```python
from build123d import *

# Parameters (mm, degrees)
EXTRUDE_1_DEPTH     = 4
EXTRUDE_2_DEPTH     = 8
CUT_EXTRUDE_1_DEPTH = 4


with BuildPart() as part:
    # Эскиз1 → Бобышка-Вытянуть1 (new body)
    with BuildSketch(Plane(origin=(0, 0, 0), x_dir=(0, 0, -1), z_dir=(1, 0, 0))):
        with BuildLine():
            Line((-7.553494652, -10.580393119), (-7.992649685, -0.342857143))
            ThreePointArc((-7.992649685, -0.342857143), (-0.171467962, 7.99816221), (8, 0))
            ThreePointArc((8, 0), (7.99816221, -0.171467962), (7.992649685, -0.342857143))
            Line((7.992649685, -0.342857143), (7.553494652, -10.580393119))
            ThreePointArc((7.553494652, -10.580393119), (11.428263628, -6.196352996), (12.988055737, -0.557142857))
            ThreePointArc((12.988055737, -0.557142857), (12.997013591, -0.278635438), (13, 0))
            ThreePointArc((13, 0), (-0.278635438, 12.997013591), (-12.988055737, -0.557142857))
            ThreePointArc((-12.988055737, -0.557142857), (-11.428263628, -6.196352996), (-7.553494652, -10.580393119))
        make_face()
        with BuildLine():
            Line((-4.727763281, -6.453545875), (-4.995406053, -0.214285714))
            ThreePointArc((-4.995406053, -0.214285714), (-0.107167476, 4.998851381), (5, 0))
            ThreePointArc((5, 0), (4.998851381, -0.107167476), (4.995406053, -0.214285714))
            Line((4.995406053, -0.214285714), (4.727763281, -6.453545875))
            ThreePointArc((4.727763281, -6.453545875), (7.056015568, -3.769966087), (7.992649685, -0.342857143))
            ThreePointArc((7.992649685, -0.342857143), (7.99816221, -0.171467962), (8, 0))
            ThreePointArc((8, 0), (-0.171467962, 7.99816221), (-7.992649685, -0.342857143))
            ThreePointArc((-7.992649685, -0.342857143), (-7.056015568, -3.769966087), (-4.727763281, -6.453545875))
        make_face()
        with BuildLine():
            Line((0, -8), (0, -5))
            ThreePointArc((0, -5), (-3.458942861, -3.610500559), (-4.995406053, -0.214285714))
            Line((-4.995406053, -0.214285714), (-4.727763281, -6.453545875))
            ThreePointArc((-4.727763281, -6.453545875), (-2.487130174, -7.603563868), (0, -8))
        make_face()
        with BuildLine():
            ThreePointArc((4.995406053, -0.214285714), (3.458942861, -3.610500559), (0, -5))
            Line((0, -5), (0, -8))
            ThreePointArc((0, -8), (2.487130174, -7.603563868), (4.727763281, -6.453545875))
            Line((4.727763281, -6.453545875), (4.995406053, -0.214285714))
        make_face()
        with BuildLine():
            ThreePointArc((4.727763281, -6.453545875), (2.487130174, -7.603563868), (0, -8))
            Line((0, -8), (0, -13))
            ThreePointArc((0, -13), (2.275699548, -12.799265274), (4.481120339, -12.203260241))
            Line((4.481120339, -12.203260241), (4.727763281, -6.453545875))
        make_face()
        with BuildLine():
            ThreePointArc((7.992649685, -0.342857143), (7.056015568, -3.769966087), (4.727763281, -6.453545875))
            Line((4.727763281, -6.453545875), (4.481120339, -12.203260241))
            ThreePointArc((4.481120339, -12.203260241), (6.071771893, -11.494937411), (7.553494652, -10.580393119))
            Line((7.553494652, -10.580393119), (7.992649685, -0.342857143))
        make_face()
        with BuildLine():
            Line((0, -13), (0, -8))
            ThreePointArc((0, -8), (-2.487130174, -7.603563868), (-4.727763281, -6.453545875))
            Line((-4.727763281, -6.453545875), (-4.481120339, -12.203260241))
            ThreePointArc((-4.481120339, -12.203260241), (-2.275699548, -12.799265274), (0, -13))
        make_face()
        with BuildLine():
            Line((-4.481120339, -12.203260241), (-4.727763281, -6.453545875))
            ThreePointArc((-4.727763281, -6.453545875), (-7.056015568, -3.769966087), (-7.992649685, -0.342857143))
            Line((-7.992649685, -0.342857143), (-7.553494652, -10.580393119))
            ThreePointArc((-7.553494652, -10.580393119), (-6.071771893, -11.494937411), (-4.481120339, -12.203260241))
        make_face()
        with BuildLine():
            Line((-3.966260715, -24.205613684), (-4.481120339, -12.203260241))
            ThreePointArc((-4.481120339, -12.203260241), (-6.071771893, -11.494937411), (-7.553494652, -10.580393119))
            Line((-7.553494652, -10.580393119), (-6.900606425, -25.80045485))
            ThreePointArc((-6.900606425, -25.80045485), (-5.491637274, -24.895945366), (-3.966260715, -24.205613684))
        make_face()
        with BuildLine():
            Line((-6.900606425, -25.80045485), (-7.553494652, -10.580393119))
            ThreePointArc((-7.553494652, -10.580393119), (-11.428263628, -6.196352996), (-12.988055737, -0.557142857))
            Line((-12.988055737, -0.557142857), (-11.489433922, -35.492857143))
            ThreePointArc((-11.489433922, -35.492857143), (-10.393943503, -30.07903074), (-6.900606425, -25.80045485))
        make_face()
        with BuildLine():
            Line((0, -23.5), (0, -13))
            ThreePointArc((0, -13), (-2.275699548, -12.799265274), (-4.481120339, -12.203260241))
            Line((-4.481120339, -12.203260241), (-3.966260715, -24.205613684))
            ThreePointArc((-3.966260715, -24.205613684), (-2.014268771, -23.677777545), (0, -23.5))
        make_face()
        with BuildLine():
            ThreePointArc((4.481120339, -12.203260241), (2.275699548, -12.799265274), (0, -13))
            Line((0, -13), (0, -23.5))
            ThreePointArc((0, -23.5), (2.014268771, -23.677777545), (3.966260715, -24.205613684))
            Line((3.966260715, -24.205613684), (4.481120339, -12.203260241))
        make_face()
        with BuildLine():
            ThreePointArc((7.553494652, -10.580393119), (6.071771893, -11.494937411), (4.481120339, -12.203260241))
            Line((4.481120339, -12.203260241), (3.966260715, -24.205613684))
            ThreePointArc((3.966260715, -24.205613684), (5.491637274, -24.895945366), (6.900606425, -25.80045485))
            Line((6.900606425, -25.80045485), (7.553494652, -10.580393119))
        make_face()
        with BuildLine():
            ThreePointArc((12.988055737, -0.557142857), (11.428263628, -6.196352996), (7.553494652, -10.580393119))
            Line((7.553494652, -10.580393119), (6.900606425, -25.80045485))
            ThreePointArc((6.900606425, -25.80045485), (10.286082196, -29.857382665), (11.5, -35))
            ThreePointArc((11.5, -35), (11.497358177, -35.246485195), (11.489433922, -35.492857143))
            Line((11.489433922, -35.492857143), (12.988055737, -0.557142857))
        make_face()
        with BuildLine():
            ThreePointArc((11.5, -35), (10.286082196, -29.857382665), (6.900606425, -25.80045485))
            Line((6.900606425, -25.80045485), (6.494027869, -35.278571429))
            ThreePointArc((6.494027869, -35.278571429), (0, -41.5), (-6.494027869, -35.278571429))
            Line((-6.494027869, -35.278571429), (-6.900606425, -25.80045485))
            ThreePointArc((-6.900606425, -25.80045485), (-10.393943503, -30.07903074), (-11.489433922, -35.492857143))
            ThreePointArc((-11.489433922, -35.492857143), (0, -46.5), (11.489433922, -35.492857143))
            ThreePointArc((11.489433922, -35.492857143), (11.497358177, -35.246485195), (11.5, -35))
        make_face()
        with BuildLine():
            ThreePointArc((6.5, -35), (5.766493566, -32.000408036), (3.731522476, -29.677806842))
            Line((3.731522476, -29.677806842), (3.496784237, -35.15))
            ThreePointArc((3.496784237, -35.15), (0, -38.5), (-3.496784237, -35.15))
            Line((-3.496784237, -35.15), (-3.731522476, -29.677806842))
            ThreePointArc((-3.731522476, -29.677806842), (-5.829460606, -32.124693225), (-6.494027869, -35.278571429))
            ThreePointArc((-6.494027869, -35.278571429), (0, -41.5), (6.494027869, -35.278571429))
            ThreePointArc((6.494027869, -35.278571429), (6.498506796, -35.139317719), (6.5, -35))
        make_face()
        with BuildLine():
            Line((-3.731522476, -29.677806842), (-3.966260715, -24.205613684))
            ThreePointArc((-3.966260715, -24.205613684), (-5.491637274, -24.895945366), (-6.900606425, -25.80045485))
            Line((-6.900606425, -25.80045485), (-6.494027869, -35.278571429))
            ThreePointArc((-6.494027869, -35.278571429), (-5.829460606, -32.124693225), (-3.731522476, -29.677806842))
        make_face()
        with BuildLine():
            Line((0, -28.5), (0, -23.5))
            ThreePointArc((0, -23.5), (-2.014268771, -23.677777545), (-3.966260715, -24.205613684))
            Line((-3.966260715, -24.205613684), (-3.731522476, -29.677806842))
            ThreePointArc((-3.731522476, -29.677806842), (-1.956494885, -28.801441477), (0, -28.5))
        make_face()
        with BuildLine():
            ThreePointArc((3.966260715, -24.205613684), (2.014268771, -23.677777545), (0, -23.5))
            Line((0, -23.5), (0, -28.5))
            ThreePointArc((0, -28.5), (1.956494885, -28.801441477), (3.731522476, -29.677806842))
            Line((3.731522476, -29.677806842), (3.966260715, -24.205613684))
        make_face()
        with BuildLine():
            Line((0, -31.5), (0, -28.5))
            ThreePointArc((0, -28.5), (-1.956494885, -28.801441477), (-3.731522476, -29.677806842))
            Line((-3.731522476, -29.677806842), (-3.496784237, -35.15))
            ThreePointArc((-3.496784237, -35.15), (-2.527350391, -32.578739997), (0, -31.5))
        make_face()
        with BuildLine():
            ThreePointArc((3.731522476, -29.677806842), (1.956494885, -28.801441477), (0, -28.5))
            Line((0, -28.5), (0, -31.5))
            ThreePointArc((0, -31.5), (2.474873734, -32.525126266), (3.5, -35))
            ThreePointArc((3.5, -35), (3.499195967, -35.075017233), (3.496784237, -35.15))
            Line((3.496784237, -35.15), (3.731522476, -29.677806842))
        make_face()
        with BuildLine():
            ThreePointArc((6.900606425, -25.80045485), (5.491637274, -24.895945366), (3.966260715, -24.205613684))
            Line((3.966260715, -24.205613684), (3.731522476, -29.677806842))
            ThreePointArc((3.731522476, -29.677806842), (5.766493566, -32.000408036), (6.5, -35))
            ThreePointArc((6.5, -35), (6.498506796, -35.139317719), (6.494027869, -35.278571429))
            Line((6.494027869, -35.278571429), (6.900606425, -25.80045485))
        make_face()
    extrude(amount=EXTRUDE_1_DEPTH)

    # Эскиз1<5> → Бобышка-Вытянуть2 (add)
    with BuildSketch(Plane(origin=(0, 0, 0), x_dir=(0, 0, -1), z_dir=(1, 0, 0))):
        with BuildLine():
            Line((-6.900606425, -25.80045485), (-7.553494652, -10.580393119))
            ThreePointArc((-7.553494652, -10.580393119), (-11.428263628, -6.196352996), (-12.988055737, -0.557142857))
            Line((-12.988055737, -0.557142857), (-11.489433922, -35.492857143))
            ThreePointArc((-11.489433922, -35.492857143), (-10.393943503, -30.07903074), (-6.900606425, -25.80045485))
        make_face()
        with BuildLine():
            Line((-6.494027869, -35.278571429), (-6.900606425, -25.80045485))
            ThreePointArc((-6.900606425, -25.80045485), (-10.393943503, -30.07903074), (-11.489433922, -35.492857143))
            ThreePointArc((-11.489433922, -35.492857143), (0, -46.5), (11.489433922, -35.492857143))
            ThreePointArc((11.489433922, -35.492857143), (11.497358177, -35.246485195), (11.5, -35))
            ThreePointArc((11.5, -35), (10.286082196, -29.857382665), (6.900606425, -25.80045485))
            Line((6.900606425, -25.80045485), (6.494027869, -35.278571429))
            ThreePointArc((6.494027869, -35.278571429), (0, -41.5), (-6.494027869, -35.278571429))
        make_face()
        with BuildLine():
            ThreePointArc((12.988055737, -0.557142857), (11.428263628, -6.196352996), (7.553494652, -10.580393119))
            Line((7.553494652, -10.580393119), (6.900606425, -25.80045485))
            ThreePointArc((6.900606425, -25.80045485), (10.286082196, -29.857382665), (11.5, -35))
            ThreePointArc((11.5, -35), (11.497358177, -35.246485195), (11.489433922, -35.492857143))
            Line((11.489433922, -35.492857143), (12.988055737, -0.557142857))
        make_face()
        with BuildLine():
            Line((-7.553494652, -10.580393119), (-7.992649685, -0.342857143))
            ThreePointArc((-7.992649685, -0.342857143), (-0.171467962, 7.99816221), (8, 0))
            ThreePointArc((8, 0), (7.99816221, -0.171467962), (7.992649685, -0.342857143))
            Line((7.992649685, -0.342857143), (7.553494652, -10.580393119))
            ThreePointArc((7.553494652, -10.580393119), (11.428263628, -6.196352996), (12.988055737, -0.557142857))
            ThreePointArc((12.988055737, -0.557142857), (12.997013591, -0.278635438), (13, 0))
            ThreePointArc((13, 0), (-0.278635438, 12.997013591), (-12.988055737, -0.557142857))
            ThreePointArc((-12.988055737, -0.557142857), (-11.428263628, -6.196352996), (-7.553494652, -10.580393119))
        make_face()
    extrude(amount=EXTRUDE_2_DEPTH)

    # Эскиз2 → Вырез-Вытянуть1 (cut)
    with BuildSketch(Plane(origin=(8, 0, 0), x_dir=(0, 0, -1), z_dir=(1, 0, 0))):
        with BuildLine():
            Line((-9.990812106, -0.428571429), (-8.49219029, -35.364285714))
            ThreePointArc((-8.49219029, -35.364285714), (0, -43.5), (8.49219029, -35.364285714))
            Line((8.49219029, -35.364285714), (9.990812106, -0.428571429))
            ThreePointArc((9.990812106, -0.428571429), (0, 10), (-9.990812106, -0.428571429))
        make_face()
    extrude(amount=-CUT_EXTRUDE_1_DEPTH, mode=Mode.SUBTRACT)


solid = part.part
```
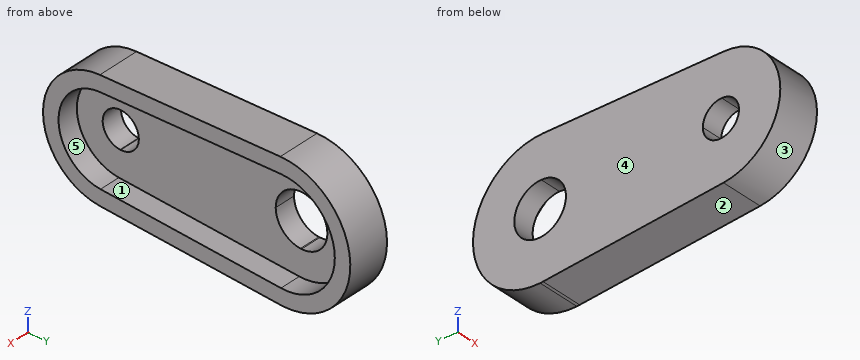
The listing builds one solid part. Answer for the finished solid, in the listing's coordinates (mm). Face numbers are marked on the shaded views. A direction names the side the tool comes from. Round coordinates to 2 decimals unless told otherwise and drop trailing zeros. Loops run counter-clockwise (first coordinate to the right, second up) from the corner with the lowest first, then second, coordinate; pieces in that order, holes last.
Q1. Section C-C, the plane x = 1.75 is taken. Determine the outline of the cut face in (y, z).
Q2. Which of the six approach directions +Z, -Z, +X, -X, +Y, -Y give full straight-line access (tool end or side, diameter ignored) to the marked faces 1 and 2?
Q3. Section D-D, the plane y = -33 is taken. Determine the outline of the cut face in (x, z).
Q4. Given pin 1 Ø2 at (x, y) = (2, -26) entering from +Z; pin 2 Ø1 at (x, z) = (4.5, -6) entering from -Y; pin 3 Ø1 at (x, y) = (3, -13.5) entering from +Z, each flat-ended and moving along its own axis, determine where each tip first touches the part or whether it passes through.
Q5. Section A-A, the plane x = 5.75 is taken. Determine the outline of the cut face in (y, z).
Q6. Find the intervals of material crossed by line 1 (X direction, y = -24.5, z = -3.5); line 2 (Z direction, x = 6.5, y = -20); line 3 (Z direction, x = 6.5, y = -4), in increasing order.
Q7. For a pull along Y with two mould halves and no side action, classify the marked faces 3, 4 and 5 as released by +Y, released by -Y, zero draft, split by the parting line, or undercut.
Q8. Section B-B, the plane y = -2 is taken. Determine the outline of the cut face in (x, z).
Completed:
1. outline: (-35.49, -11.49) - (-0.56, -12.99) arc R13 ccw (long way) to (-0.56, 12.99) - (-35.49, 11.49) arc R11.5 ccw to start; hole circle Ø7 at (-35, 0); hole (-0.21, -5) arc R5 ccw to (0, -5) arc R5 ccw (long way) to start
2. face 1: +X
2. face 2: -Z, +X, -X, -Y
3. outline: (0, -11.6) - (8, -11.6) - (8, -8.59) - (4, -8.59) - (4, -2.87) - (0, -2.87) - close; (0, 2.87) - (4, 2.87) - (4, 8.59) - (8, 8.59) - (8, 11.6) - (0, 11.6) - close
4. pin 1: stops at z = 11.94
4. pin 2: stops at y = -45.1
4. pin 3: stops at z = 12.45
5. outline: (-35.49, -11.49) - (-0.56, -12.99) arc R13 ccw (long way) to (-0.56, 12.99) - (-35.49, 11.49) arc R11.5 ccw to start; hole (-35.36, -8.49) - (-0.43, -9.99) arc R10 ccw (long way) to (-0.43, 9.99) - (-35.36, 8.49) arc R8.5 ccw to start
6. line 1: x = 0 to 4
6. line 2: z = -12.15 to -9.15, 9.15 to 12.15
6. line 3: z = -12.84 to -9.84, 9.84 to 12.84
7. face 3: released by -Y
7. face 4: zero draft
7. face 5: undercut
8. outline: (0, -12.93) - (8, -12.93) - (8, -9.92) - (4, -9.92) - (4, -4.58) - (0, -4.58) - close; (0, 4.58) - (4, 4.58) - (4, 9.92) - (8, 9.92) - (8, 12.93) - (0, 12.93) - close
